```python
from build123d import *

# Parameters (mm, degrees)
SKETCH1_R               = 4
BOSS_EXTRUDE1_DEPTH     = 1.5
CUT_EXTRUDE1_DEPTH      = 6.852349955
CUT_EXTRUDE1_DEPTH_BACK = 6.852349955
SKETCH2_R               = 3.25
SKETCH4_W               = 0.5
SKETCH4_H               = 2
FILLET1_R               = 0.5


with BuildPart() as part:
    # Sketch1 → Boss-Extrude1 (new, symmetric)
    with BuildSketch(Plane(origin=(0, 0, 0), x_dir=(1, 0, 0), z_dir=(0, 1, 0))):
        with Locations(Location((0, 0, 0), (0, 0, 270))):
            Circle(SKETCH1_R)
    extrude(amount=BOSS_EXTRUDE1_DEPTH, both=True)

    # Sketch2 → Cut-Extrude1 (cut, two sides: drawn at the far end of the back side and taken through both)
    with BuildSketch(Plane(origin=(0, 0, 0), x_dir=(1, 0, 0), z_dir=(0, 1, 0)).offset(-CUT_EXTRUDE1_DEPTH_BACK)):
        with Locations(Location((0, 0, 0), (0, 0, 270))):
            Circle(SKETCH2_R)
    extrude(amount=CUT_EXTRUDE1_DEPTH + CUT_EXTRUDE1_DEPTH_BACK, mode=Mode.SUBTRACT)

    # Sketch4 → Cut-Revolve1 (revolve, cut)
    with BuildSketch(Plane(origin=(0, 0, 0), x_dir=(0, 0, -1), z_dir=(1, 0, 0))):
        with Locations((-3.75, 0)):
            Rectangle(SKETCH4_W, SKETCH4_H)
    revolve(axis=Axis((0, 1.1156594, 0), (0, -1, 0)), mode=Mode.SUBTRACT)

    # Fillet1
    fillet1_edges = [part.edges().sort_by_distance(p)[0] for p in [
        (0, -1.5, -4),
        (0, 1.5, -4),
    ]]
    fillet(fillet1_edges, radius=FILLET1_R - 0.0001)  # a hair under: the kernel refuses the full size


solid = part.part
```
Work out the finished part from the listing and answer in its coordinate system (mm). Round coordinates to 2 decimals unless told otherwise and drop trailing zeros. Write each loop counter-clockwise with the first axis right and the second up, starting at its lowest first coordinate (ties: lowest second). Pieces come first, ordered by that corner, then holes.
1) Flat-ended cylindrical pins translate along their axes: P1, Ø1, axis at x = -1.5, z = 1, coming from the +Y side; P2, Ø1.5, axis at y = -1, z = -1, coming from the +X side. Find the tip coordinate at first contact, or state that the pin passes through.
2) Consider probe 1 along X at (y, z) = (0.7, 0); probe 2 along X at (y, z) = (-0.55, -1). Determine where each line is inside the solid, lowest interval first.
3) Determine the mould class of faces 1 (the face through (1.341, 0.014, 3.233)), 2 (the face through (-1.978, -0.021, -2.579)) for opening direction Y: pulls with the +Y half, pulls with the -Y half, needs draft (parallel to the pull), parting line crosses it, or undercut.
4) A cutting plane is placed at C-C on y = 0.15. Determine the outline of the cut face in (x, z).
5) A cutting plane is placed at D-D on y = -1.2. Determine the outline of the cut face in (x, z).
Entries:
1. P1: passes through
1. P2: stops at x = 3.99
2. probe 1: x = -3.5 to -3.25, 3.25 to 3.5
2. probe 2: x = -3.35 to -3.09, 3.09 to 3.35
3. face 1: undercut
3. face 2: needs draft
4. outline: circle Ø7 at (0, 0); hole circle Ø6.5 at (0, 0)
5. outline: circle Ø7.92 at (0, 0); hole circle Ø6.5 at (0, 0)
